Here's how the part is built. I have some questions about the finished solid (model axes, mm). Face numbers are marked on the shaded views. A direction names the side the tool comes from. Coordinates: 2 decimals unless noted, no trailing zeros. Loops run counter-clockwise (first coordinate to the right, second up) from the corner with the lowest first, then second, coordinate; pieces in that order, holes last.
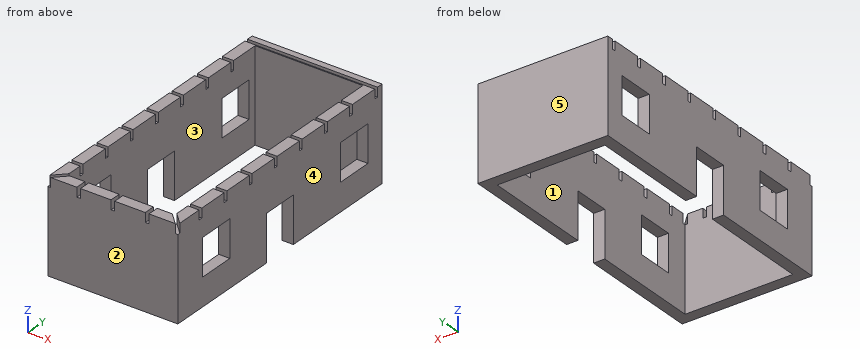
```python
from build123d import *

# Parameters (mm, degrees)
F0_W      = 70
F0_H      = 150
F0_W_2    = 58
F0_H_2    = 138
F1_DEPTH  = 50
F2_W      = 2
F2_H      = 6
F3_DEPTH  = 5
F4_W      = 2
F4_H      = 6
F5_DEPTH  = 5
F7_DEPTH  = 5
F8_W      = 20
F8_H      = 20
F8_W_2    = 19.828947
F8_H_2    = 25
F9_DEPTH  = 200
F10_DEPTH = 25


with BuildPart() as f1:
    # F0 (on Top) → F1 (new body)
    with BuildSketch(Plane.XY):
        Rectangle(F0_W, F0_H)
        Rectangle(F0_W_2, F0_H_2, mode=Mode.SUBTRACT)
    extrude(amount=F1_DEPTH)

    # F2 (on face) → F3 (cut)
    with BuildSketch(Plane.XY.offset(50)):
        with Locations((0, -72)):
            Rectangle(F2_W, F2_H)
        Polygon((-34.292893, -75.707107), (-28.292893, -69.707107), (-27.585786, -69), (-29, -67.585786), (-29.707107, -68.292893), (-35.707107, -74.292893), align=None)
        Polygon((27.585786, -69), (28.292893, -69.707107), (33.585786, -75), (35, -75), (35, -73.585786), (29.707107, -68.292893), (29, -67.585786), align=None)
    extrude(amount=-F3_DEPTH, mode=Mode.SUBTRACT)

    # F4 (on face) → F5 (cut)
    with BuildSketch(Plane.XY.offset(50)):
        with Locations((-18.44, -72)):
            Rectangle(F4_W, F4_H)
        with Locations((18.44, -72)):
            Rectangle(F4_W, F4_H)
    extrude(amount=-F5_DEPTH, mode=Mode.SUBTRACT)

    # F6 (on face) → F7 (cut)
    with BuildSketch(Plane.XY.offset(50)):
        Polygon((29, -59.435786), (35, -59.435786), (35, -57.435786), (29, -57.435786), (-66.520862, -57.435786), (-66.520862, -59.435786), align=None)
        Polygon((35, -40.995786), (35, -38.995786), (29, -38.995786), (-40.70507, -38.995786), (-40.70507, -40.995786), (29, -40.995786), align=None)
        Polygon((35, -22.555786), (35, -20.555786), (29, -20.555786), (-41.178755, -20.555786), (-41.178755, -22.555786), (29, -22.555786), align=None)
        Polygon((35, -4.115786), (35, -2.115786), (29, -2.115786), (-41.403655, -2.115786), (-41.403655, -4.115786), (29, -4.115786), align=None)
        Polygon((35, 14.324214), (35, 16.324214), (29, 16.324214), (-43.992728, 16.324214), (-43.992728, 14.324214), (29, 14.324214), align=None)
        Polygon((35, 32.764214), (35, 34.764214), (29, 34.764214), (-43.992728, 34.764214), (-43.992728, 32.764214), (29, 32.764214), align=None)
        Polygon((35, 51.204214), (35, 53.204214), (29, 53.204214), (-39.611217, 53.204214), (-39.611217, 51.204214), (29, 51.204214), align=None)
        Polygon((29, 69.644214), (35, 69.644214), (35, 71.644214), (29, 71.644214), (-35, 71.644214), (-35, 69.644214), align=None)
    extrude(amount=-F7_DEPTH, mode=Mode.SUBTRACT)

    # F8 (on face) → F9 (cut)
    with BuildSketch(Plane(origin=(-35, 0, 0), x_dir=(0, -1, 0), z_dir=(-1, 0, 0))):
        with Locations((-54.592106, 25)):
            Rectangle(F8_W, F8_H)
        with Locations((46.825401, 25)):
            Rectangle(F8_W, F8_H)
        with Locations((0.085527, 12.5)):
            Rectangle(F8_W_2, F8_H_2)
    extrude(amount=-F9_DEPTH, mode=Mode.SUBTRACT)

    # F8 (on face) → F10 (cut)
    with BuildSketch(Plane(origin=(-35, 0, 0), x_dir=(0, -1, 0), z_dir=(-1, 0, 0))):
        with Locations((-54.592106, 25)):
            Rectangle(F8_W, F8_H)
        with Locations((46.825401, 25)):
            Rectangle(F8_W, F8_H)
        with Locations((0.085527, 12.5)):
            Rectangle(F8_W_2, F8_H_2)
    extrude(amount=-F10_DEPTH, mode=Mode.SUBTRACT)


solid = f1.part
```
1. For pin 1 (0.6 mm diameter, centred on x = -32, y = 15, fed in from +Z); pin 2 (2 mm diameter, centred on x = 32, y = -21.5, fed in from +Z); pin 3 (1.5 mm diameter, centred on y = -3, z = 22.5, fed in from +X), each with a flat end and sliding along its axis, tell me the tip position at first contact or that it passes through.
2. We'd pull the mould along Y, two halves only. Please class the marked faces 3, 4 and 5: +Y half, -Y half, draft (parallel to the pull), parting line (faces both ways), or undercut.
3. I want a section at C-C (x = 15.5). Please give me the cut outline in (y, z), then the cut area to 3 significant figures.
4. I want a section at D-D (z = 28). Please give me the cut outline in (x, y), then the cut area to 3 significant figures.
5. I want a section at A-A (z = 7.5). Please give me the cut outline in (x, y).
6. On a 3-axis mill with a long thin cutter (end or side, diameter ignored), from which of +Z, -Z, +X, -X, +Y, -Y can I reach the whole of each face in a straight line? I mean the marked faces 1 and 2. Say none if no direction works.
7. I need wall thicknesses on line 1 along Y through (x, z) = (32, 32); line 2 along Y through (x, z) = (-21.5, 41); line 3 along Y through (x, z) = (32.5, 5.5). Which ranges of each line are inside material? Lowest first, please.
8. I want a section at B-B (y = -63). Please give me the cut outline in (x, z).
Response values:
1. pin 1: stops at z = 45
1. pin 2: stops at z = 50
1. pin 3: passes through
2. face 3: undercut
2. face 4: draft
2. face 5: +Y half
3. outline: (-75, 0) - (-69, 0) - (-69, 50) - (-75, 50) - close; (69, 0) - (75, 0) - (75, 50) - (71.64, 50) - (71.64, 45) - (69.64, 45) - (69.64, 50) - (69, 50) - close
3. area: 590 mm2
4. outline: (-35, -75) - (35, -75) - (35, -56.83) - (29, -56.83) - (29, -69) - (-29, -69) - (-29, -56.83) - (-35, -56.83) - close; (-35, -36.83) - (-29, -36.83) - (-29, 44.59) - (-35, 44.59) - close; (-35, 64.59) - (-29, 64.59) - (-29, 69) - (29, 69) - (29, 64.59) - (35, 64.59) - (35, 75) - (-35, 75) - close; (29, -36.83) - (35, -36.83) - (35, 44.59) - (29, 44.59) - close
4. area: 2,020 mm2
5. outline: (-35, -75) - (35, -75) - (35, -10) - (29, -10) - (29, -69) - (-29, -69) - (-29, -10) - (-35, -10) - close; (-35, 9.83) - (-29, 9.83) - (-29, 69) - (29, 69) - (29, 9.83) - (35, 9.83) - (35, 75) - (-35, 75) - close
6. face 1: +Z, -Z
6. face 2: +Z, -Z, +X, -X, -Y
7. line 1: y = -75 to -56.83, -36.83 to 44.59, 64.59 to 75
7. line 2: y = -75 to -69, 69 to 75
7. line 3: y = -75 to -10, 9.83 to 75
8. outline: (-35, 0) - (-29, 0) - (-29, 50) - (-35, 50) - close; (29, 0) - (35, 0) - (35, 50) - (29, 50) - close
